Geometry: see drawing. Coordinates: mm, zero at the bounding-box minimum. A direction names the side the tool comes from. Round coordinates to 2 decimals unless told otherwise and drop trailing zeros. Order: outer loops, then holes, each group sorted by start corner. A loop starts at its lowest first (then second) coordinate and runs counter-clockwise, first axis right, second up. Notation, with made-up numbers: (83, 48.25) -> (131, 48.25) arc R8 ccw to (131, 61.25) -> close; hole circle Ø9 at (-1.75, -19.5). An arc over 180 degrees is marked (long way). One line per item, written item: value. Start each with the question number.
1) Section D-D (x = 2). Return the cut outline in (y, z).
2) Mould query, pull axis Y, two halves, no side actions, for the marked faces 1, 2, 3 and 4. Classes: pulls with the +Y half, pulls with the -Y half, needs draft (parallel to the pull), parting line crosses it, or undercut.
3) Reachability of the marked faces 5 and 6 from +Z, -Z, +X, -X, +Y, -Y: full face, straight path, thin tool, end or side. Return the list, or none.
4) Ray query, L1, parallel to X at y = 11.5, z = 1.1; L2, parallel to Y at x = 11.75, z = 7; L3, parallel to Y at x = 13, z = 3.3. Return the intervals inside material, ascending.
5) Section A-A (x = 5). Return the cut outline in (y, z).
6) Section C-C (y = 11.5). Return the cut outline in (x, z).
7) Section B-B (z = 5). Return the cut outline in (x, y).
8) Pin query (flat end, axial travel): P1, Ø5.5, axis at x = 4, y = 11, coming from the +Z side; P2, Ø4, axis at x = 13, y = 11.5, coming from the +Z side; P3, Ø3, axis at x = 13, y = 11.5, coming from the +Z side. Return the tip coordinate at first contact, or that it passes through.
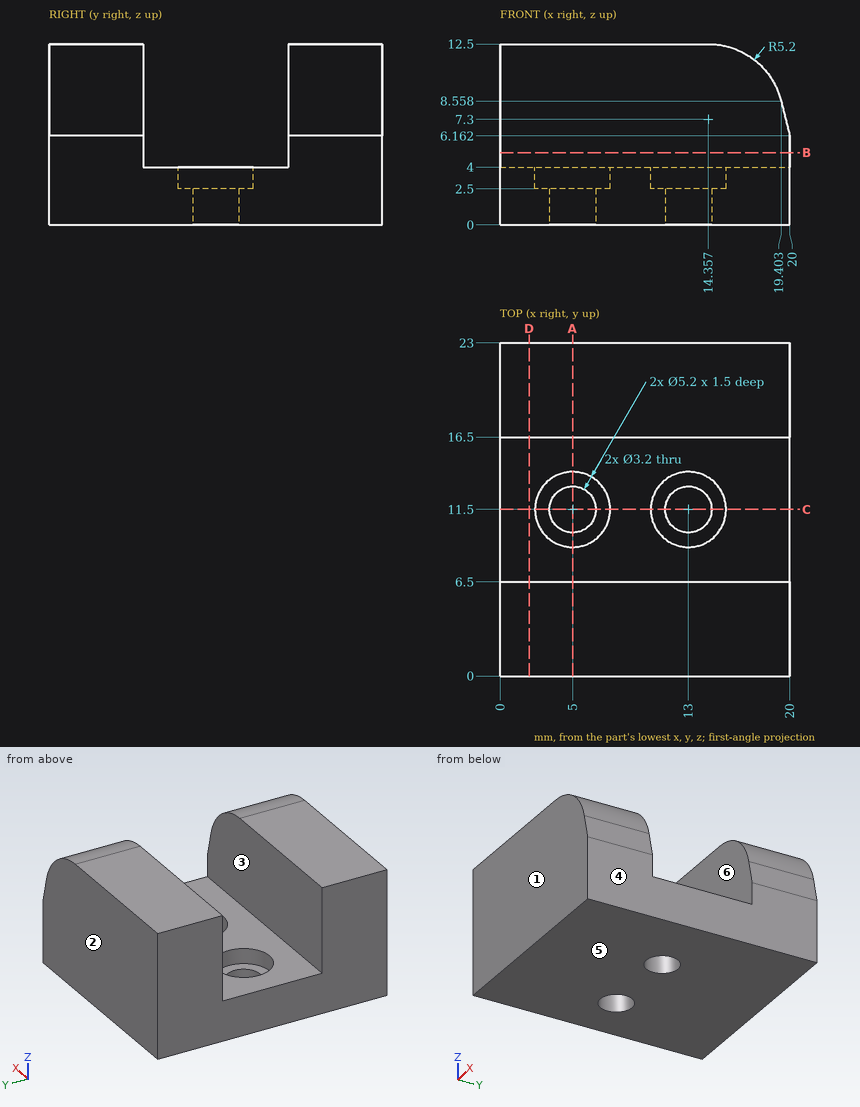
Findings:
1. outline: (0, 0) -> (23, 0) -> (23, 12.5) -> (16.5, 12.5) -> (16.5, 4) -> (6.5, 4) -> (6.5, 12.5) -> (0, 12.5) -> close
2. face 1: pulls with the -Y half
2. face 2: pulls with the +Y half
2. face 3: undercut
2. face 4: needs draft
3. face 5: -Z, +X, -X, +Y, -Y
3. face 6: +Z, +X, -X
4. L1: 0 to 3.4, 6.6 to 11.4, 14.6 to 20
4. L2: 0 to 6.5, 16.5 to 23
4. L3: 0 to 8.9, 14.1 to 23
5. outline: (0, 0) -> (9.9, 0) -> (9.9, 2.5) -> (8.9, 2.5) -> (8.9, 4) -> (6.5, 4) -> (6.5, 12.5) -> (0, 12.5) -> close; (13.1, 0) -> (23, 0) -> (23, 12.5) -> (16.5, 12.5) -> (16.5, 4) -> (14.1, 4) -> (14.1, 2.5) -> (13.1, 2.5) -> close
6. outline: (0, 0) -> (3.4, 0) -> (3.4, 2.5) -> (2.4, 2.5) -> (2.4, 4) -> (0, 4) -> close; (6.6, 0) -> (11.4, 0) -> (11.4, 2.5) -> (10.4, 2.5) -> (10.4, 4) -> (7.6, 4) -> (7.6, 2.5) -> (6.6, 2.5) -> close; (14.6, 0) -> (20, 0) -> (20, 4) -> (15.6, 4) -> (15.6, 2.5) -> (14.6, 2.5) -> close
7. outline: (0, 0) -> (20, 0) -> (20, 6.5) -> (0, 6.5) -> close; (0, 16.5) -> (20, 16.5) -> (20, 23) -> (0, 23) -> close
8. P1: z = 4
8. P2: z = 2.5
8. P3: through
